Source: CAD feature listing. Evaluate the final solid. Frame: model axes, mm. A direction names the side the tool comes from. Round coordinates to 2 decimals unless told otherwise and drop trailing zeros. Loops run counter-clockwise (first coordinate to the right, second up) from the corner with the lowest first, then second, coordinate; pieces in that order, holes last. Notation, with made-up numbers: (-2, 66.25) -> (53, 66.25) arc R24 ccw to (53, 102.25) -> close; hole circle Ø1 at (32.25, -13). An arc over 180 degrees is marked (long way). Put each result on its own line as item: value. Start each with the question number.
1. Contact query for flat-ended pins moving along their axis: pin 1 (1.8 mm diameter, centred on x = 0, z = 0, fed in from -Y); pin 2 (0.6 mm diameter, centred on x = 0, z = 3, fed in from -Y); pin 3 (4 mm diameter, centred on y = 19.5, z = 2.5, fed in from -X). Output: stop coordinate, or through.
2. Draft query along X for faces 1 (the cylindrical face through (2.58, 7.58, 4.05)), 2 (the flat face through (2.3, 0, -0.1)), 3 (the cylindrical face through (0, 1, -2)). Return one class per face: pulls with the +X half, pulls with the -X half, needs draft (parallel to the pull), parting line crosses it, or undercut.
3. Cut plane A-A (z = 0). Return the cut outline in (x, y), then the cut area to 3 significant figures.
4. Material intervals for L1, parallel to Z at x = 0, y = 17.5; L2, parallel to Y at x = -3.75, z = -1; L3, parallel to Y at x = 3.75, z = -3.5, sorted ascending.
5. Cut plane B-B (y = 9). Return the cut outline in (x, z).
6. Set-up query: faces 4 (the cylindrical face through (-3, 19, 0)), 5 (the flat face through (1.3, 22.6, 0)), 6 (the flat face through (0.4, 1, 3)). Return all of +Z, -Z, +X, -X, +Y, -Y with unobstructed straight access to the full face (end or side cutting, diameter ignored); none if empty.
```python
from build123d import *

# Parameters (mm, degrees)
CROQUIS7_R              = 5.3
SALIENTE_EXTRUIR1_DEPTH = 2
CORTAR_EXTRUIR1_START   = 7.6
CROQUIS3_R              = 1.15
CORTAR_EXTRUIR1_DEPTH   = 7.8
CROQUIS4_R              = 2
CORTAR_EXTRUIR2_DEPTH   = 2.6
CORTAR_EXTRUIR4_DEPTH   = 2


with BuildPart() as part:
    # Croquis1 → Revolución2 (revolve)
    with BuildSketch(Plane.XY):
        Polygon((4.8, 15), (3, 15), (3, 22.6), (0, 22.6), (0, 0), (4.8, 0), align=None)
    revolve(axis=Axis((0, 55, 0), (0, -1, 0)))

    # Croquis7 → Saliente-Extruir1 (add)
    with BuildSketch(Plane(origin=(0, 15, 0), x_dir=(1, 0, 0), z_dir=(0, 1, 0))):
        Circle(CROQUIS7_R)
    saliente_extruir1 = extrude(amount=-SALIENTE_EXTRUIR1_DEPTH)

    # Croquis3 → Cortar-Extruir1 (cut)
    with BuildSketch(Plane(origin=(0, 15, 0), x_dir=(1, 0, 0), z_dir=(0, 1, 0)).offset(CORTAR_EXTRUIR1_START)):
        Circle(CROQUIS3_R)
    extrude(amount=-CORTAR_EXTRUIR1_DEPTH, mode=Mode.SUBTRACT)

    # Croquis8 → Cortar-Revolución2 (revolve, cut)
    with BuildSketch(Plane(origin=(0, 0, 0), x_dir=(0, 0, -1), z_dir=(1, 0, 0))):
        with BuildLine():
            Line((5.3, 15), (5.3, 13))
            Line((5.3, 13), (4.8, 13))
            ThreePointArc((4.8, 13), (4.872810183, 14.044297454), (5.3, 15))
        make_face()
    cortar_revoluci_n2 = revolve(axis=Axis((0, 55, 0), (0, -1, 0)), mode=Mode.SUBTRACT)

    # Simetría1: Saliente-Extruir1, Cortar-Revolución2 across plane
    add(saliente_extruir1.mirror(Plane(origin=(0, 7.5, 0), x_dir=(0, 0, 1), z_dir=(0, -1, 0))))
    add(cortar_revoluci_n2.mirror(Plane(origin=(0, 7.5, 0), x_dir=(0, 0, 1), z_dir=(0, -1, 0))), mode=Mode.SUBTRACT)

    # Croquis4 → Cortar-Extruir2 (cut)
    with BuildSketch(Plane.XZ):
        Circle(CROQUIS4_R)
    extrude(amount=-CORTAR_EXTRUIR2_DEPTH, mode=Mode.SUBTRACT)

    # Croquis9 → Cortar-Extruir4 (cut)
    with BuildSketch(Plane.XZ):
        Polygon((-0.4, 3.2), (0, 4), (0.4, 3.2), (0.4, 2.4), (-0.4, 2.4), align=None)
    extrude(amount=-CORTAR_EXTRUIR4_DEPTH, mode=Mode.SUBTRACT)


solid = part.part
```
Solution:
1. pin 1: stops at y = 2.6
1. pin 2: stops at y = 2
1. pin 3: stops at x = -2.96
2. face 1: parting line crosses it
2. face 2: needs draft
2. face 3: undercut
3. outline: (-5.3, 0) -> (-2, 0) -> (-2, 2.6) -> (2, 2.6) -> (2, 0) -> (5.3, 0) arc R3 cw to (4.8, 2) -> (4.8, 13) arc R3 cw to (5.3, 15) -> (3, 15) -> (3, 22.6) -> (1.15, 22.6) -> (1.15, 14.8) -> (-1.15, 14.8) -> (-1.15, 22.6) -> (-3, 22.6) -> (-3, 15) -> (-5.3, 15) arc R3 cw to (-4.8, 13) -> (-4.8, 2) arc R3 cw to start
3. area: 162 mm^2
4. L1: z = -3 to -1.15, 1.15 to 3
4. L2: y = 0 to 15
4. L3: y = 0 to 0.28, 14.72 to 15
5. outline: circle Ø9.6 at (0, 0)
6. face 4: +Y
6. face 5: +Z, -Z, +X, -X, +Y
6. face 6: -Y
